from build123d import *

# Parameters (mm, degrees)
SKETCH_1_R               = 20
EXTRUDE_1_DEPTH          = 35
SKETCH_3_R               = 30
EXTRUDE_2_DEPTH          = 1
EXTRUDE_START            = -1
SKETCH_4_R               = 30
EXTRUDE_3_DEPTH          = 1
CUT_EXTRUDE_2_DEPTH      = 56
CUT_EXTRUDE_2_DEPTH_BACK = 56
SKETCH_5_W               = 1
SKETCH_5_H               = 13
EXTRUDE_4_DEPTH          = 21.5
CUT_EXTRUDE_3_REACH      = 50.5
PATTERN_CIRCULAR_2_COUNT = 10
CUT_EXTRUDE_5_DEPTH      = 56
CUT_EXTRUDE_5_DEPTH_BACK = 56


with BuildPart() as part:
    # Sketch 1 → Extrude 1 (new body)
    with BuildSketch(Plane.XY):
        Circle(SKETCH_1_R)
    extrude(amount=EXTRUDE_1_DEPTH)

    # Sketch 3 → Extrude 2 (add)
    with BuildSketch(Plane.XY.offset(35)):
        Circle(SKETCH_3_R)
    extrude(amount=-EXTRUDE_2_DEPTH)

    # Sketch 4 → Extrude 3 (add)
    with BuildSketch(Plane(origin=(0, 0, 0), x_dir=(-1, 0, 0), z_dir=(0, 0, -1)).offset(EXTRUDE_START)):
        with Locations(Location((0, 0, 0), (0, 0, 180))):
            Circle(SKETCH_4_R)
    extrude(amount=EXTRUDE_3_DEPTH)

    # Sketch 2 → Cut-Extrude 2 (cut, two sides: drawn at the far end of the back side and taken through both)
    with BuildSketch(Plane.XY.offset(35).offset(-CUT_EXTRUDE_2_DEPTH_BACK)):
        with BuildLine():
            Line((-1.944865034, 1.8), (1.944865034, 1.8))
            ThreePointArc((1.944865034, 1.8), (2.65, 0), (1.944865034, -1.8))
            Line((1.944865034, -1.8), (-1.944865034, -1.8))
            ThreePointArc((-1.944865034, -1.8), (-2.65, 0), (-1.944865034, 1.8))
        make_face()
    extrude(amount=CUT_EXTRUDE_2_DEPTH + CUT_EXTRUDE_2_DEPTH_BACK, mode=Mode.SUBTRACT)

    # Sketch 5 → Extrude 4 (add)
    with BuildSketch(Plane(origin=(0, 0, 0), x_dir=(1, 0, 0), z_dir=(0, 1, 0))):
        with Locations((0, -17)):
            Rectangle(SKETCH_5_W, SKETCH_5_H)
    extrude_4 = extrude(amount=EXTRUDE_4_DEPTH)

    # Sketch 6 → Cut-Extrude 3 (cut, up to next)
    with BuildSketch(Plane.XY.offset(23.5), mode=Mode.PRIVATE) as cut_extrude_3_sk1:
        Polygon((-0.5, 19.993749023), (0, 21.5), (-0.5, 21.5), align=None)
    cut_extrude_3_tool1 = extrude(cut_extrude_3_sk1.sketch, amount=-CUT_EXTRUDE_3_REACH, mode=Mode.PRIVATE) & part.part
    # Sketch 6 → Cut-Extrude 3 (cut, up to next)
    with BuildSketch(Plane.XY.offset(23.5), mode=Mode.PRIVATE) as cut_extrude_3_sk2:
        Polygon((0.5, 21.5), (0, 21.5), (0.5, 19.993749023), align=None)
    cut_extrude_3_tool2 = extrude(cut_extrude_3_sk2.sketch, amount=-CUT_EXTRUDE_3_REACH, mode=Mode.PRIVATE) & part.part
    cut_extrude_3_1 = cut_extrude_3_tool1.solids().sort_by_distance((-0.333333, 20.997916, 23.5))[0]
    add(cut_extrude_3_1, mode=Mode.SUBTRACT)
    cut_extrude_3_2 = cut_extrude_3_tool2.solids().sort_by_distance((0.333333, 20.997916, 23.5))[0]
    add(cut_extrude_3_2, mode=Mode.SUBTRACT)
    cut_extrude_3 = cut_extrude_3_1 + cut_extrude_3_2  # Cut-Extrude 3 as one shape, for the pattern or mirror that repeats it

    # Pattern Circular 2: Extrude 4, Cut-Extrude 3 ×10 about axis
    pattern_circular_2_axis = Axis((0, 0, 0), (0, 0, 1))
    add([extrude_4.rotate(pattern_circular_2_axis, i * 360 / PATTERN_CIRCULAR_2_COUNT) for i in range(1, PATTERN_CIRCULAR_2_COUNT)])
    add([cut_extrude_3.rotate(pattern_circular_2_axis, i * 360 / PATTERN_CIRCULAR_2_COUNT) for i in range(1, PATTERN_CIRCULAR_2_COUNT)], mode=Mode.SUBTRACT)

    # Sketch 8 → Cut-Extrude 5 (cut, two sides: drawn at the far end of the back side and taken through both)
    with BuildSketch(Plane.XY.offset(35).offset(-CUT_EXTRUDE_5_DEPTH_BACK)):
        with BuildLine():
            ThreePointArc((-1.944865034, -1.8), (-2.65, 0), (-1.944865034, 1.8))
            Line((-1.944865034, 1.8), (1.944865034, 1.8))
            ThreePointArc((1.944865034, 1.8), (2.65, 0), (1.944865034, -1.8))
            Line((1.944865034, -1.8), (-1.944865034, -1.8))
        make_face()
    extrude(amount=CUT_EXTRUDE_5_DEPTH + CUT_EXTRUDE_5_DEPTH_BACK, mode=Mode.SUBTRACT)


solid = part.part
Design review of the part built by this model. Coordinates are the model's own, in mm. A direction names the side the tool comes from. Give positions to 0.01 mm unless a question says otherwise; leave off trailing zeros. Order: outer loops, then holes, each group sorted by start corner. A loop starts at its lowest first (then second) coordinate and runs counter-clockwise, first axis right, second up. Notation, with made-up numbers: (-29, -38.75) - (29, -38.75) arc R32 ccw to (29, -0.75) - close; hole circle Ø2 at (-29.75, -13.75). An arc over 180 degrees is marked (long way). Write item = value, one per line. Start each with the question number.
Q1. Clearance check with flat-ended pins moving along their axes: pin 1 Ø4 at (x, z) = (4.5, 31.5) entering from -Y; pin 2 Ø8 at (y, z) = (7, 19) entering from +X; pin 3 Ø8 at (y, z) = (-8, 24) entering from -X. State where each tip first meets the part, or that it passes through.
Q2. Tool access review of faces 1 (the face through (6, -20, 34)), 2 (the face through (0, -1.8, 17)), 3 (the face through (-12.394, 16.627, 17.091)): name each direction out of +Z, -Z, +X, -X, +Y, -Y from which nothing blocks a thin tool from reaching the whole face with its end or side.
Q3. We need section A-A on y = 0. State the section outline as (x, z) points, plus the area to 3 significant figures.
Q4. We need section D-D on x = -8.5. State the section outline as (y, z) points.
Q5. To check wall thickness, follow L1, parallel to Z at x = 12, y = -27; L2, parallel to Y at x = 0, z = 7.5; L3, parallel to Y at x = 2, z = 33. State the ranges of each line that lie inside material, in increasing order. Write a range as from..to.
Q6. Mouldability with a two-part tool opening along Y and no side actions: class faces 4 (the face through (6, 20, 1)), 5 (the face through (0.247, 20.757, 17.091)), 6 (the face through (12.4, 16.65, 17.09)) as released by +Y, released by -Y, zero draft, split by the parting line, or undercut.
Q7. We need section C-C on z = 3. State the section outline as (x, y) points, plus the area to 3 significant figures.
Working result:
q1.pin_1 = -19.84
q1.pin_2 = 20.45
q1.pin_3 = -20.45
q2.face_1 = none
q2.face_2 = +Z, -Z
q2.face_3 = -X
q3.outline = (-30, 0) - (-2.65, 0) - (-2.65, 35) - (-30, 35) - (-30, 34) - (-20, 34) - (-20, 1) - (-30, 1) - close; (2.65, 0) - (30, 0) - (30, 1) - (20, 1) - (20, 34) - (30, 34) - (30, 35) - (2.65, 35) - close
q3.area = 1,250 mm²
q4.outline = (-28.77, 0) - (28.77, 0) - (28.77, 1) - (18.1, 1) - (18.1, 34) - (28.77, 34) - (28.77, 35) - (-28.77, 35) - (-28.77, 34) - (-18.1, 34) - (-18.1, 1) - (-28.77, 1) - close
q5.L1 = 0..1, 34..35
q5.L2 = -20..-1.8, 1.8..20
q5.L3 = -19.9..-1.74, 1.74..19.9
q6.face_4 = zero draft
q6.face_5 = released by +Y
q6.face_6 = undercut
q7.outline = circle Ø40 at (0, 0); hole (-1.94, -1.8) - (1.94, -1.8) arc R2.65 ccw to (1.94, 1.8) - (-1.94, 1.8) arc R2.65 ccw to start
q7.area = 1,240 mm²
